Here's how the part is built. I have some questions about the finished solid (model axes, mm). Face numbers are marked on the shaded views. Coordinates: 2 decimals unless noted, no trailing zeros. Write each loop counter-clockwise with the first axis right and the second up, starting at its lowest first coordinate (ties: lowest second). Pieces come first, ordered by that corner, then holes. Notation, with made-up numbers: (15.5, 88.25) -> (62.5, 88.25) arc R11 cw to (62.5, 104.25) -> close; hole circle Ø8 at (-26.5, 5.25). An arc over 180 degrees is marked (long way). Use a Markdown table: item, result. Add a question column.
Item 1: If I drill on line 1 along X through (y, z) = (1.2, -7.5); line 2 along Z through (x, y) = (-19.5, 1); line 3 along X through (y, z) = (4.85, -7.5), over which ranges is the centre line in solid material (lowest first)? Write a range as from..to.
Item 2: Imagine slicing it at D-D, the plane y = 5.2. Write out the boundary of the cut face in (x, z).
Item 3: Imagine slicing it at C-C, the plane z = -7. Write out the boundary of the cut face in (x, y), and give its area (3 significant figures).
Item 4: Will these pins go through, and if not, where does the flat tip stop? pin 1 Ø1.5 at (x, y) = (-13.5, 2) entering from +Z; pin 2 Ø3 at (x, z) = (-20, -7.5) entering from +Y; pin 3 Ø1.7 at (x, z) = (-21, -8) entering from -Y; pin 4 Ø4.5 at (x, z) = (-6, -7.5) entering from +Y.
Item 5: Imagine slicing it at A-A, the plane x = -20. Write out the boundary of the cut face in (y, z).
Item 6: If we mould it in two halves opening along X, with no side actions, what happens to the marked faces 1, 2 and 3? For each: pulls with the +X half, pulls with the -X half, needs draft (parallel to the pull), parting line crosses it, or undercut.
Item 7: Imagine slicing it at B-B, the plane y = 0.8. Write out the boundary of the cut face in (x, z), and give its area (3 significant figures).
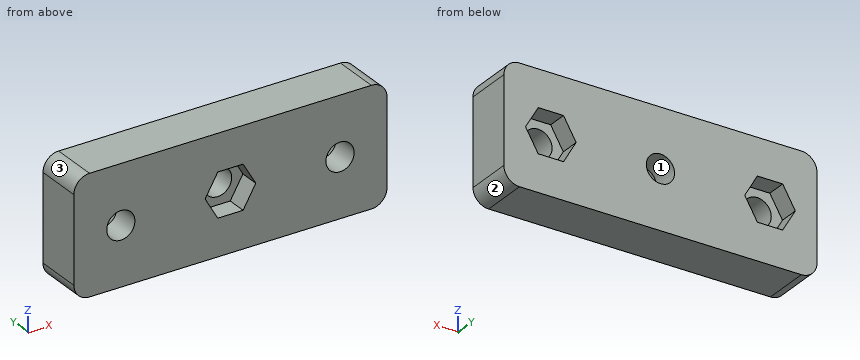
Autodesk Inventor part; units mm, degrees
ref_plane "YZ Plane" through (0, 0, 0) normal (1, 0, 0) x (0, 1, 0)
ref_plane "XZ Plane" through (0, 0, 0) normal (0, 1, 0) x (-1, 0, 0)
ref_plane "XY Plane" through (0, 0, 0) normal (0, 0, 1) x (1, 0, 0)
sketch "Sketch1" plane through (0, 0, 0) normal (0, 1, 0) x (-1, 0, 0)
  line L0 (0, 0) -> (40, 0)
  line L1 (40, 0) -> (40, -15)
  line L2 (40, -15) -> (0, -15)
  line L3 (0, -15) -> (0, 0)
  dimension "d0" = 40
  dimension "d1" = 15
extrude "Extrusion1" add sketch "Sketch1" along normal blind 6
fillet "Fillet1" radius 2 4 edges at (0, 3, 0) (0, 3, -15) (-40, 3, -15) (-40, 3, 0)
ref_plane "Work Plane1" through (-20, 0, -2) normal (1, 0, 0) x (0, 0, -1)
sketch "Sketch2" plane through (0, 6, 0) normal (0, 1, 0) x (1, 0, 0)
  circle A0 centre (-6, 7.5) radius 1.8
  point P0 (0, 0)
  dimension "d9" = 3.6
extrude "Extrusion3" cut sketch "Sketch2" against normal blind 6
sketch "Sketch4" plane through (0, 6, 0) normal (0, 1, 0) x (1, 0, 0)
  circle A0 centre (-6, 7.5) radius 1.8
  line L0 (-7.6166, 4.7) -> (-9.2332, 7.5)
  line L1 (-9.2332, 7.5) -> (-7.6166, 10.3)
  line L2 (-7.6166, 10.3) -> (-4.3834, 10.3)
  line L3 (-4.3834, 10.3) -> (-2.7668, 7.5)
  line L4 (-2.7668, 7.5) -> (-4.3834, 4.7)
  line L5 (-4.3834, 4.7) -> (-7.6166, 4.7)
  point P0 (0, 0)
  point P1 (-6, 4.7)
extrude "Extrusion4" cut sketch "Sketch4" against normal blind 2.5
sketch "Sketch5" plane through (0, 6, 0) normal (0, 1, 0) x (1, 0, 0)
  circle A0 centre (-20, 7.5) radius 1.8
  point P0 (0, 0)
  dimension "d15" = 3.6
extrude "Extrusion5" cut sketch "Sketch5" against normal blind 6
sketch "Sketch6" plane through (0, 0, 0) normal (0, -1, 0) x (1, 0, 0)
  circle A0 centre (-20, -7.5) radius 1.8
  line L0 (-21.6166, -10.3) -> (-23.2332, -7.5)
  line L1 (-23.2332, -7.5) -> (-21.6166, -4.7)
  line L2 (-21.6166, -4.7) -> (-18.3834, -4.7)
  line L3 (-18.3834, -4.7) -> (-16.7668, -7.5)
  line L4 (-16.7668, -7.5) -> (-18.3834, -10.3)
  line L5 (-18.3834, -10.3) -> (-21.6166, -10.3)
  point P0 (0, 0)
  point P1 (-20, -10.3)
extrude "Extrusion6" cut sketch "Sketch6" against normal blind 2.5
mirror "Mirror1" about plane through (-20, 0, -2) normal (1, 0, 0) of "Extrusion3"
mirror "Mirror2" about plane through (-20, 0, -2) normal (1, 0, 0) of "Extrusion4"
properties part number "shaft pusher top"
Ans:
| question | item | result |
|---|---|---|
| 1 | line 1 | x = -40..-35.8, -32.2..-23.23, -16.77..-7.8, -4.2..0 |
| 1 | line 2 | z = -15..-10.3, -4.7..0 |
| 1 | line 3 | x = -40..-37.23, -30.77..-21.8, -18.2..-9.23, -2.77..0 |
| 2 | outline | (-40, -13) arc R2 ccw to (-38, -15) -> (-2, -15) arc R2 ccw to (0, -13) -> (0, -2) arc R2 ccw to (-2, 0) -> (-38, 0) arc R2 ccw to (-40, -2) -> close; hole (-37.23, -7.5) -> (-35.62, -10.3) -> (-32.38, -10.3) -> (-30.77, -7.5) -> (-32.38, -4.7) -> (-35.62, -4.7) -> close; hole circle Ø3.6 at (-20, -7.5); hole (-9.23, -7.5) -> (-7.62, -10.3) -> (-4.38, -10.3) -> (-2.77, -7.5) -> (-4.38, -4.7) -> (-7.62, -4.7) -> close |
| 3 | outline | (-40, 0) -> (-35.73, 0) -> (-35.73, 3.5) -> (-36.94, 3.5) -> (-36.94, 6) -> (-40, 6) -> close; (-32.27, 0) -> (-22.94, 0) -> (-22.94, 2.5) -> (-21.73, 2.5) -> (-21.73, 6) -> (-31.06, 6) -> (-31.06, 3.5) -> (-32.27, 3.5) -> close; (-18.27, 2.5) -> (-17.06, 2.5) -> (-17.06, 0) -> (-7.73, 0) -> (-7.73, 3.5) -> (-8.94, 3.5) -> (-8.94, 6) -> (-18.27, 6) -> close; (-4.27, 0) -> (0, 0) -> (0, 6) -> (-3.06, 6) -> (-3.06, 3.5) -> (-4.27, 3.5) -> close |
| 3 | area | 160 mm^2 |
| 4 | pin 1 | stops at z = 0 |
| 4 | pin 2 | passes through |
| 4 | pin 3 | stops at y = 2.5 |
| 4 | pin 4 | stops at y = 3.5 |
| 5 | outline | (0, -15) -> (6, -15) -> (6, -9.3) -> (2.5, -9.3) -> (2.5, -10.3) -> (0, -10.3) -> close; (0, -4.7) -> (2.5, -4.7) -> (2.5, -5.7) -> (6, -5.7) -> (6, 0) -> (0, 0) -> close |
| 6 | face 1 | undercut |
| 6 | face 2 | pulls with the +X half |
| 6 | face 3 | pulls with the -X half |
| 7 | outline | (-40, -13) arc R2 ccw to (-38, -15) -> (-2, -15) arc R2 ccw to (0, -13) -> (0, -2) arc R2 ccw to (-2, 0) -> (-38, 0) arc R2 ccw to (-40, -2) -> close; hole circle Ø3.6 at (-34, -7.5); hole (-23.23, -7.5) -> (-21.62, -10.3) -> (-18.38, -10.3) -> (-16.77, -7.5) -> (-18.38, -4.7) -> (-21.62, -4.7) -> close; hole circle Ø3.6 at (-6, -7.5) |
| 7 | area | 549 mm^2 |
